```python
from build123d import *

# Parameters (mm, degrees)
F0_R     = 14.2875
F0_R_2   = 11.0236
F1_DEPTH = 6.35


with BuildPart() as f1:
    # F0 (on Front) → F1 (new body)
    with BuildSketch(Plane.XZ):
        with BuildLine():
            ThreePointArc((0.052564, 41.773122), (-7.567375, 41.80347), (-11.403627, 35.219583))
            Line((-11.403627, 35.219583), (0.052564, 41.773122))
        make_face()
        Polygon((0.052564, 41.773122), (-11.403627, 35.219583), (-11.456191, 22.021461), (-8.534462, 20.319048), (-0.052564, 15.376878), (8.586806, 20.319048), (11.403627, 21.930417), (11.456191, 35.128539), align=None)
        Polygon((-8.757622, 23.565183), (-8.71744, 33.654415), (0.040182, 38.664231), (8.757622, 33.584817), (8.71744, 23.495585), (-0.040182, 18.485769), align=None, mode=Mode.SUBTRACT)
        with BuildLine():
            Line((-11.456191, 22.021461), (-11.403627, 35.219583))
            ThreePointArc((-11.403627, 35.219583), (-15.239879, 28.635696), (-11.456191, 22.021461))
        make_face()
        with BuildLine():
            ThreePointArc((11.456191, 35.128539), (7.672504, 41.742775), (0.052564, 41.773122))
            Line((0.052564, 41.773122), (11.456191, 35.128539))
        make_face()
        with BuildLine():
            ThreePointArc((11.403627, 21.930417), (15.239879, 28.514304), (11.456191, 35.128539))
            Line((11.456191, 35.128539), (11.403627, 21.930417))
        make_face()
        with BuildLine():
            Line((-0.052564, 15.376878), (-8.534462, 20.319048))
            ThreePointArc((-8.534462, 20.319048), (-12.800156, 16.577999), (-13.126936, 10.913654))
            ThreePointArc((-13.126936, 10.913654), (-22.380073, 5.66998), (-18.992298, -4.411669))
            Line((-18.992298, -4.411669), (-13.290484, -7.733961))
            Line((-13.290484, -7.733961), (-13.316767, -14.333022))
            ThreePointArc((-13.316767, -14.333022), (-7.854296, -20.65549), (0, -17.805539))
            ThreePointArc((0, -17.805539), (7.832001, -20.409484), (13.316767, -14.241978))
            Line((13.316767, -14.241978), (13.343049, -7.642917))
            Line((13.343049, -7.642917), (19.071144, -4.366147))
            ThreePointArc((19.071144, -4.366147), (21.571506, 5.766311), (12.492773, 10.913654))
            ThreePointArc((12.492773, 10.913654), (12.206621, 16.30857), (8.586806, 20.319048))
            Line((8.586806, 20.319048), (-0.052564, 15.376878))
        make_face()
        Circle(F0_R, mode=Mode.SUBTRACT)
        Polygon((-13.290484, -7.733961), (-18.992298, -4.411669), (-24.694112, -1.089378), (-36.150303, -7.642917), (-36.202867, -20.841039), (-24.79924, -27.485622), (-13.343049, -20.932083), (-13.316767, -14.333022), align=None)
        Polygon((-33.464115, -9.208085), (-24.706494, -4.198269), (-15.989054, -9.277683), (-16.029236, -19.366915), (-24.786858, -24.376731), (-33.504298, -19.297317), align=None, mode=Mode.SUBTRACT)
        with BuildLine():
            Line((-36.150303, -7.642917), (-24.694112, -1.089378))
            ThreePointArc((-24.694112, -1.089378), (-32.314051, -1.05903), (-36.150303, -7.642917))
        make_face()
        Polygon((24.79924, -1.089378), (19.071144, -4.366147), (13.343049, -7.642917), (13.316767, -14.241978), (13.290484, -20.841039), (24.694112, -27.485622), (36.150303, -20.932083), (36.202867, -7.733961), align=None)
        Polygon((24.706494, -24.376731), (15.989054, -19.297317), (16.029236, -9.208085), (24.786858, -4.198269), (33.504298, -9.277683), (33.464115, -19.366915), align=None, mode=Mode.SUBTRACT)
        with BuildLine():
            Line((-36.202867, -20.841039), (-36.150303, -7.642917))
            ThreePointArc((-36.150303, -7.642917), (-39.986555, -14.226804), (-36.202867, -20.841039))
        make_face()
        with BuildLine():
            ThreePointArc((36.202867, -7.733961), (32.41918, -1.119725), (24.79924, -1.089378))
            Line((24.79924, -1.089378), (36.202867, -7.733961))
        make_face()
        with BuildLine():
            Line((-24.79924, -27.485622), (-36.202867, -20.841039))
            ThreePointArc((-36.202867, -20.841039), (-32.41918, -27.455275), (-24.79924, -27.485622))
        make_face()
        with BuildLine():
            ThreePointArc((-24.79924, -27.485622), (-17.1793, -27.51597), (-13.343049, -20.932083))
            Line((-13.343049, -20.932083), (-24.79924, -27.485622))
        make_face()
        with BuildLine():
            ThreePointArc((36.150303, -20.932083), (39.986555, -14.348196), (36.202867, -7.733961))
            Line((36.202867, -7.733961), (36.150303, -20.932083))
        make_face()
        with BuildLine():
            Line((24.694112, -27.485622), (13.290484, -20.841039))
            ThreePointArc((13.290484, -20.841039), (17.074172, -27.455275), (24.694112, -27.485622))
        make_face()
        with BuildLine():
            ThreePointArc((24.694112, -27.485622), (32.314051, -27.51597), (36.150303, -20.932083))
            Line((36.150303, -20.932083), (24.694112, -27.485622))
        make_face()
        Circle(F0_R)
        Circle(F0_R_2, mode=Mode.SUBTRACT)
    extrude(amount=F1_DEPTH)


solid = f1.part
```
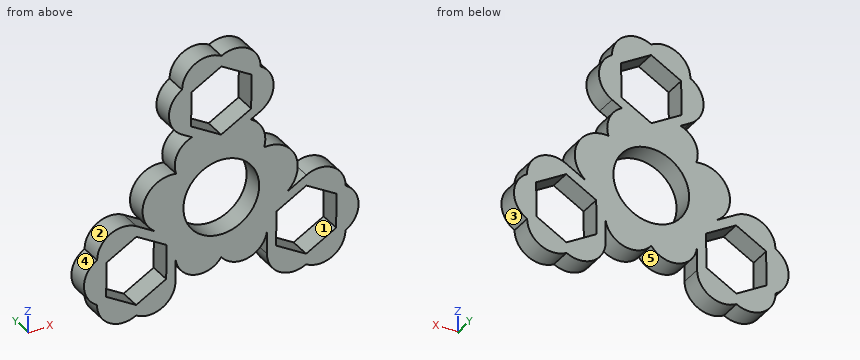
Geometry check sheet. Reference: the model listing, model coordinates, mm. Face numbers are marked on the shaded views. A direction names the side the tool comes from. Give positions to 0.01 mm unless a question says otherwise; leave off trailing zeros. Write each loop counter-clockwise with the first axis right and the second up, starting at its lowest first coordinate (ties: lowest second). Pieces come first, ordered by that corner, then holes. Notation, with made-up numbers: (76, -3) - (101, -3) arc R34 cw to (101, 30) - close; hole circle Ø2 at (49.25, 17). An arc over 180 degrees is marked (long way). Use a Markdown table: item, result.
Q1. Draft check along X on the marked faces 3, 4 and 5. Enter one of: pulls with the +X half, pulls with the -X half, needs draft (parallel to the pull), parting line crosses it, or undercut.
Computed:
| item | result |
|---|---|
| face 3 | pulls with the +X half |
| face 4 | pulls with the -X half |
| face 5 | undercut |
Q2. Section check B-B, the plane x = -20. Enter the section's corners in (y, z), then the cut area to 3 significant figures.
Computed:
| item | result |
|---|---|
| outline | (-6.35, -28.46) - (0, -28.46) - (0, -21.64) - (-6.35, -21.64) - close; (-6.35, -6.94) - (0, -6.94) - (0, -3.82) - (-6.35, -3.82) - close; (-6.35, -3.67) - (0, -3.67) - (0, 9.04) - (-6.35, 9.04) - close |
| area | 144 mm² |
Q3. Set-up check for the marked faces 1 and 2: record each of +Z, -Z, +X, -X, +Y, -Y from which the full face is reachable in a straight line by a thin tool's end or side.
Computed:
| item | result |
|---|---|
| face 1 | +Y, -Y |
| face 2 | +Z, +Y, -Y |
Q4. Section check A-A, the plane z = 27.5. Enter the section's corners in (x, y).
Computed:
| item | result |
|---|---|
| outline | (-15.16, -6.35) - (-8.74, -6.35) - (-8.74, 0) - (-15.16, 0) - close; (8.73, -6.35) - (15.17, -6.35) - (15.17, 0) - (8.73, 0) - close |
Q5. Section check C-C, the plane z = -23. Enter the section's corners in (x, y).
Computed:
| item | result |
|---|---|
| outline | (-35.9, -6.35) - (-27.15, -6.35) - (-27.15, 0) - (-35.9, 0) - close; (-22.38, -6.35) - (-13.64, -6.35) - (-13.64, 0) - (-22.38, 0) - close; (13.59, -6.35) - (22.34, -6.35) - (22.34, 0) - (13.59, 0) - close; (27.11, -6.35) - (35.86, -6.35) - (35.86, 0) - (27.11, 0) - close |
Q6. Go/stop test with flat-tipped pins: P1, Ø1, axis at y = -2, z = 26.5, coming from the +X side; P2, Ø1.5, axis at y = -5.5, z = 19.5, coming from the -X side; P3, Ø1.5, axis at x = 22, z = -8, coming from the -Y side. Record where each tip stops, or that it passes through.
Computed:
| item | result |
|---|---|
| P1 | stops at x = 15.08 |
| P2 | stops at x = -11.18 |
| P3 | passes through |
Q7. Section check D-D, the plane z = 4. Enter the section's corners in (x, y), then the cut area to 3 significant figures.
Computed:
| item | result |
|---|---|
| outline | (-22.83, -6.35) - (-10.27, -6.35) - (-10.27, 0) - (-22.83, 0) - close; (10.27, -6.35) - (22.12, -6.35) - (22.12, 0) - (10.27, 0) - close |
| area | 155 mm² |
Q8. Thickness scan on L1, parallel to X at y = -1, z = -14; L2, parallel to X at y = -4.5, z = -19; L3, parallel to Z at x = -6.5, y = -5. Record the ranges inside material, lowest first. Write a range as [from, to].
Computed:
| item | result |
|---|---|
| L1 | x = [-39.98, -33.48], [-16.01, 16.01], [33.49, 39.98] |
| L2 | x = [-38.33, -33.5], [-16.03, -13.34], [-10.93, -1.07], [1.18, 10.6], [13.3, 15.99], [33.47, 38.38] |
| L3 | z = [-20.88, -8.9], [8.9, 22.25], [34.92, 42.31] |
